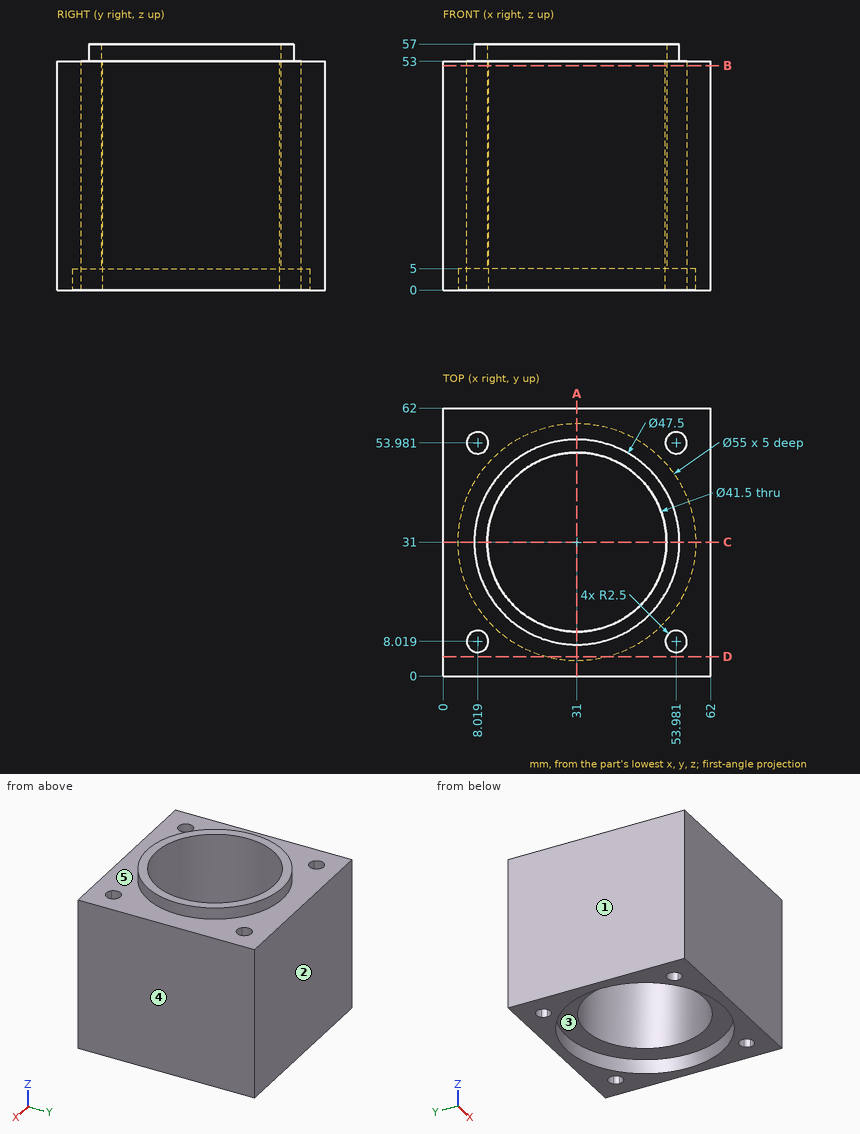
Geometry check sheet. Reference: drawing and pictorial views, mm from the part's lowest x, y, z. A direction names the side the tool comes from. Coordinates: 2 decimals unless noted, no trailing zeros. Order: outer loops, then holes, each group sorted by start corner. A loop starts at its lowest first (then second) coordinate and runs counter-clockwise, first axis right, second up. Notation, with made-up numbers: (50.5, 20.25) -> (69.5, 20.25) arc R20 ccw to (69.5, 55.25) -> close; hole circle Ø3 at (89.5, 87). An arc over 180 degrees is marked (long way). Put each result on its own line as item: value. Start each with the question number.
1) Cross-section at D-D (y = 4.5). Enter the section's corners in (x, z).
2) Cross-section at B-B (z = 52). Enter the section's corners in (x, y), plus the area to 3 significant figures.
3) Material ranges on L1, parallel to X at y = 31, z = 19; L2, parallel to Y at x = 31, z = 2.25, recorded low to high.
4) Release check for a two-part mould opening along X. For the marked faces 1, 2 and 3 record: pulls with the +X half, pulls with the -X half, needs draft (parallel to the pull), parting line crosses it, or undercut.
5) Cross-section at A-A (x = 31). Enter the section's corners in (y, z), plus the area to 3 significant figures.
6) Go/stop test with flat-tipped pins: pin 1 (10 mm diameter, centred on x = 28.5, z = 14.5, fed in from -Y); pin 2 (16.5 mm diameter, centred on x = 41, y = 30.5, fed in from -Z). Record where each tip stops, or that it passes through.
7) Tool access check on the marked faces 4 and 5. Record the directions out of +Z, -Z, +X, -X, +Y, -Y that give a thin tool (end or side, any length) a straight path to the whole face; none if there is none.
Geometry check:
1. outline: (0, 0) -> (23.65, 0) -> (23.65, 5) -> (38.35, 5) -> (38.35, 0) -> (62, 0) -> (62, 53) -> (0, 53) -> close
2. outline: (0, 0) -> (62, 0) -> (62, 62) -> (0, 62) -> close; hole circle Ø5 at (8.02, 8.02); hole circle Ø5 at (8.02, 53.98); hole circle Ø41.5 at (31, 31); hole circle Ø5 at (53.98, 8.02); hole circle Ø5 at (53.98, 53.98)
2. area: 2,410 mm^2
3. L1: x = 0 to 10.25, 51.75 to 62
3. L2: y = 0 to 3.5, 58.5 to 62
4. face 1: pulls with the -X half
4. face 2: needs draft
4. face 3: undercut
5. outline: (0, 0) -> (3.5, 0) -> (3.5, 5) -> (10.25, 5) -> (10.25, 57) -> (7.25, 57) -> (7.25, 53) -> (0, 53) -> close; (51.75, 5) -> (58.5, 5) -> (58.5, 0) -> (62, 0) -> (62, 53) -> (54.75, 53) -> (54.75, 57) -> (51.75, 57) -> close
5. area: 1,040 mm^2
6. pin 1: stops at y = 0
6. pin 2: passes through
7. face 4: +Z, -Z, +X, +Y, -Y
7. face 5: +Z
